from build123d import *

# Parameters (mm, degrees)
SKETCH1_W            = 100
SKETCH1_H            = 50
BOSS_EXTRUDE1_DEPTH  = 2
SKETCH2_W            = 73.5
SKETCH2_H            = 1.6
BOSS_EXTRUDE2_DEPTH  = 9
LPATTERN2_COUNT      = 3
LPATTERN2_PITCH      = 1.65
SKETCH3_W            = 18.8
SKETCH3_H            = 12
BOSS_EXTRUDE3_DEPTH  = 4.6
SKETCH4_W            = 48.5
SKETCH4_H            = 2.3
BOSS_EXTRUDE4_DEPTH  = 11
SKETCH5_W            = 54.8
SKETCH5_H            = 27.6
BOSS_EXTRUDE5_DEPTH  = 1.5
SKETCH6_W            = 8.5
SKETCH6_H            = 5
BOSS_EXTRUDE6_DEPTH  = 1.5
SKETCH7_R            = 4
BOSS_EXTRUDE7_DEPTH  = 3
SKETCH8_W            = 2.5
SKETCH8_H            = 10.5
SKETCH8_H_2          = 5.25
BOSS_EXTRUDE8_DEPTH  = 10
SKETCH9_W            = 24.5
SKETCH9_H            = 18.75
BOSS_EXTRUDE9_DEPTH  = 1.5
SKETCH10_W           = 2.3
SKETCH10_H           = 10.5
BOSS_EXTRUDE10_DEPTH = 9.5


with BuildPart() as part:
    # Sketch1 → Boss-Extrude1 (new body)
    with BuildSketch(Plane(origin=(0, 0, 0), x_dir=(1, 0, 0), z_dir=(0, 1, 0))):
        Rectangle(SKETCH1_W, SKETCH1_H)
    extrude(amount=BOSS_EXTRUDE1_DEPTH)

    # Sketch2 → Boss-Extrude2 (add)
    with BuildSketch(Plane(origin=(0, 2, 0), x_dir=(1, 0, 0), z_dir=(0, 1, 0))):
        with Locations((-3.25, -24.2)):
            Rectangle(SKETCH2_W, SKETCH2_H)
    boss_extrude2 = extrude(amount=BOSS_EXTRUDE2_DEPTH)

    # LPattern2: Boss-Extrude2 ×3
    with Locations(*[(0, 0, -i * LPATTERN2_PITCH) for i in range(1, LPATTERN2_COUNT)]):
        add(boss_extrude2)

    # Sketch3 → Boss-Extrude3 (add)
    with BuildSketch(Plane.XZ):
        with Locations((55.4, 0)):
            Rectangle(SKETCH3_W, SKETCH3_H)
    extrude(amount=BOSS_EXTRUDE3_DEPTH)

    # Sketch4 → Boss-Extrude4 (add)
    with BuildSketch(Plane(origin=(0, 2, 0), x_dir=(1, 0, 0), z_dir=(0, 1, 0))):
        with Locations((-25.75, -10.15)):
            Rectangle(SKETCH4_W, SKETCH4_H)
        with Locations((-25.75, 15.15)):
            Rectangle(SKETCH4_W, SKETCH4_H)
    extrude(amount=BOSS_EXTRUDE4_DEPTH)

    # Sketch5 → Boss-Extrude5 (add)
    with BuildSketch(Plane(origin=(0, 13, 0), x_dir=(1, 0, 0), z_dir=(0, 1, 0))):
        with Locations((-25.6, 2.5)):
            Rectangle(SKETCH5_W, SKETCH5_H)
    extrude(amount=BOSS_EXTRUDE5_DEPTH)

    # Sketch6 → Boss-Extrude6 (add)
    with BuildSketch(Plane(origin=(0, 14.5, 0), x_dir=(1, 0, 0), z_dir=(0, 1, 0))):
        with Locations((1.05, 2.5)):
            Rectangle(SKETCH6_W, SKETCH6_H)
    extrude(amount=BOSS_EXTRUDE6_DEPTH)

    # Sketch7 → Boss-Extrude7 (add)
    with BuildSketch(Plane(origin=(5.3, 0, 0), x_dir=(0, 0, -1), z_dir=(1, 0, 0))):
        with Locations((2.5, 15.179402112)):
            Circle(SKETCH7_R)
    extrude(amount=BOSS_EXTRUDE7_DEPTH)

    # Sketch8 → Boss-Extrude8 (add)
    with BuildSketch(Plane(origin=(0, 2, 0), x_dir=(1, 0, 0), z_dir=(0, 1, 0))):
        with Locations((25.05, -5.75)):
            Rectangle(SKETCH8_W, SKETCH8_H)
        with Locations((21.25, 5.125)):
            Rectangle(SKETCH8_W, SKETCH8_H_2)
    extrude(amount=BOSS_EXTRUDE8_DEPTH)

    # Sketch9 → Boss-Extrude9 (add)
    with BuildSketch(Plane(origin=(0, 12, 0), x_dir=(1, 0, 0), z_dir=(0, 1, 0))):
        with Locations((32.25, -1.625)):
            Rectangle(SKETCH9_W, SKETCH9_H)
    extrude(amount=BOSS_EXTRUDE9_DEPTH)

    # Sketch10 → Boss-Extrude10 (add)
    with BuildSketch(Plane(origin=(0, 13.5, 0), x_dir=(1, 0, 0), z_dir=(0, 1, 0))):
        with Locations((40.35, -5.25)):
            Rectangle(SKETCH10_W, SKETCH10_H)
    extrude(amount=BOSS_EXTRUDE10_DEPTH)


solid = part.part
Verification items for the finished model (mm, model axes). A direction names the side the tool comes from. Coordinates: 2 decimals unless noted, no trailing zeros. Write each loop counter-clockwise with the first axis right and the second up, starting at its lowest first coordinate (ties: lowest second). Pieces come first, ordered by that corner, then holes. Notation, with made-up numbers: M 56,71 L 62,71 A22 ccw 62,95 Z; hole C -2.75,-17.75 d6. An arc over 180 degrees is marked long. One line per question, with ' | ' between items.
1) Sectioned sample at C-C on z = -21.5. Record the cut outline in (x, y), then the cut area to 3 significant figures.
Solutions:
outline: M -50,0 L 50,0 L 50,2 L -50,2 Z | area: 200 mm^2
2) Material ranges on L1, parallel to Y at x = 28, z = 8; L2, parallel to Y at x = -40.5, z = 6; L3, parallel to Y at x = 47.5, z = -8, recorded low to high.
Solutions:
L1: 0 to 2, 12 to 13.5 | L2: 0 to 2, 13 to 14.5 | L3: 0 to 2
3) Depth check by flat-ended pin: pin 1 Ø0.8 at (x, z) = (-1, 24.5) entering from +Y; pin 2 Ø0.5 at (y, z) = (6, 22.5) entering from +X; pin 3 Ø1.2 at (x, y) = (1, 15) entering from +Z. Enter the tip coordinate at first touch or a pass-through.
Solutions:
pin 1: y = 11 | pin 2: x = 33.5 | pin 3: z = 11.3
4) Release check for a two-part mould opening along Y. For faces 1 (the face through (55, -2, -6)), 2 (the face through (-1.5, 7, 10)), 3 (the face through (55, -4.6, 0)) record: +Y half, -Y half, draft (parallel to the pull), parting line (faces both ways), or undercut.
Solutions:
face 1: draft | face 2: undercut | face 3: -Y half
5) Sectioned sample at B-B on y = 4. Record the cut outline in (x, z).
Solutions:
outline: M -50,-16.3 L -1.5,-16.3 L -1.5,-14 L -50,-14 Z; M -50,9 L -1.5,9 L -1.5,11.3 L -50,11.3 Z; M -40,20.1 L 33.5,20.1 L 33.5,21.7 L -40,21.7 Z; M -40,21.75 L 33.5,21.75 L 33.5,23.35 L -40,23.35 Z; M -40,23.4 L 33.5,23.4 L 33.5,25 L -40,25 Z; M 20,-7.75 L 22.5,-7.75 L 22.5,-2.5 L 20,-2.5 Z; M 23.8,0.5 L 26.3,0.5 L 26.3,11 L 23.8,11 Z
6) Access from +Z, -Z, +X, -X, +Y, -Y to the whole of each face (thin tool, end or side, straight path). Record for faces 4 (the face through (40, 18, 0)), 5 (the face through (46, -2, 0)), 6 (the face through (23.8, 7, 6)), 7 (the face through (55, -2, 6)).
Solutions:
face 4: -Z, +X, +Y | face 5: +Z, -Z, -X, -Y | face 6: -Z | face 7: +Z, +X, -X, -Y
7) Sectioned sample at A-A on x = -42. Record the cut outline in (y, z).
Solutions:
outline: M 0,-25 L 2,-25 L 2,-16.3 L 14.5,-16.3 L 14.5,11.3 L 2,11.3 L 2,25 L 0,25 Z; hole M 2,-14 L 13,-14 L 13,9 L 2,9 Z
